Read the model definition and answer for the solid it produces. Units are mm, in the model's axes. A direction names the side the tool comes from. Coordinates: 2 decimals unless noted, no trailing zeros. Write each loop counter-clockwise with the first axis right and the second up, starting at its lowest first coordinate (ties: lowest second). Pieces come first, ordered by that corner, then holes. Notation, with made-up numbers: (74.5, 89) -> (90.5, 89) arc R12 ccw to (90.5, 103) -> close; hole circle Ø10 at (24, 57). An arc over 180 degrees is marked (long way). One line per item, written item: value. Start each with the question number.
from build123d import *

# Parameters (mm, degrees)
F0_W     = 25
F0_H     = 17
F1_DEPTH = 5.5
F3_DEPTH = 25
F5_DEPTH = 32.501
F7_DEPTH = 5.5
F9_DEPTH = 5.501


with BuildPart() as f1:
    # F0 (on Top) → F1 (new body)
    with BuildSketch(Plane.XY):
        with BuildLine():
            Line((-15.5, -24.3527164447), (15.5, -24.3527164447))
            Line((15.5, -24.3527164447), (15.5, 11.6472835553))
            Line((15.5, 11.6472835553), (16.5, 11.6472835553))
            ThreePointArc((16.5, 11.6472835553), (16.8535533906, 11.7937301647), (17, 12.1472835553))
            Line((17, 12.1472835553), (17, 16.843435978))
            ThreePointArc((17, 16.843435978), (16.8977774789, 17.6198931134), (16.5980762114, 18.343435978))
            Line((16.5980762114, 18.343435978), (15.1841674029, 20.7923978715))
            ThreePointArc((15.1841674029, 20.7923978715), (14.4494876631, 21.1305094363), (13.8862846459, 20.5500991403))
            Line((13.8862846459, 20.5500991403), (12.678607693, 12.7943144757))
            ThreePointArc((12.678607693, 12.7943144757), (12.5447185816, 11.6438227741), (12.5, 10.4864301451))
            Line((12.5, 10.4864301451), (12.5, 0.6472835553))
            ThreePointArc((12.5, 0.6472835553), (11.9142135624, -0.766930007), (10.5, -1.3527164447))
            Line((10.5, -1.3527164447), (5.7, -1.3527164447))
            ThreePointArc((5.7, -1.3527164447), (4.2857864376, -0.766930007), (3.7, 0.6472835553))
            Line((3.7, 0.6472835553), (3.7, 18.6472835553))
            ThreePointArc((3.7, 18.6472835553), (3.8975072906, 19.7178136174), (4.4640230758, 20.6473853514))
            Line((4.4640230758, 20.6473853514), (5.7959697488, 22.1364105755))
            ThreePointArc((5.7959697488, 22.1364105755), (6.362485534, 23.0659823095), (6.5599928246, 24.1365123716))
            Line((6.5599928246, 24.1365123716), (6.5599928246, 25.3001695988))
            ThreePointArc((6.5599928246, 25.3001695988), (6.2513345408, 25.762109365), (5.706439434, 25.6537229894))
            Line((5.706439434, 25.6537229894), (2.0786796564, 22.0259632118))
            ThreePointArc((2.0786796564, 22.0259632118), (1.4283614025, 21.0526931653), (1.2, 19.9046428682))
            Line((1.2, 19.9046428682), (1.2, -2.3527164447))
            Line((1.2, -2.3527164447), (-1.2, -2.3527164447))
            Line((-1.2, -2.3527164447), (-1.2, 20.1675462621))
            ThreePointArc((-1.2, 20.1675462621), (-1.4283614025, 21.3155965592), (-2.0786796564, 22.2888666056))
            Line((-2.0786796564, 22.2888666056), (-5.706439434, 25.9166263832))
            ThreePointArc((-5.706439434, 25.9166263832), (-6.2513345408, 26.0250127589), (-6.5599928246, 25.5630729926))
            Line((-6.5599928246, 25.5630729926), (-6.5599928246, 24.1365123716))
            ThreePointArc((-6.5599928246, 24.1365123716), (-6.362485534, 23.0659823095), (-5.7959697488, 22.1364105755))
            Line((-5.7959697488, 22.1364105755), (-4.4640230758, 20.6473853514))
            ThreePointArc((-4.4640230758, 20.6473853514), (-3.8975072906, 19.7178136174), (-3.7, 18.6472835553))
            Line((-3.7, 18.6472835553), (-3.7, 0.6472835553))
            ThreePointArc((-3.7, 0.6472835553), (-4.2857864376, -0.766930007), (-5.7, -1.3527164447))
            Line((-5.7, -1.3527164447), (-10.5, -1.3527164447))
            ThreePointArc((-10.5, -1.3527164447), (-11.9142135624, -0.766930007), (-12.5, 0.6472835553))
            Line((-12.5, 0.6472835553), (-12.5, 10.4864301451))
            ThreePointArc((-12.5, 10.4864301451), (-12.5447185816, 11.6438227741), (-12.678607693, 12.7943144757))
            Line((-12.678607693, 12.7943144757), (-13.8862846459, 20.5500991403))
            ThreePointArc((-13.8862846459, 20.5500991403), (-14.4494876631, 21.1305094363), (-15.1841674029, 20.7923978715))
            Line((-15.1841674029, 20.7923978715), (-16.5980762114, 18.343435978))
            ThreePointArc((-16.5980762114, 18.343435978), (-16.8977774789, 17.6198931134), (-17, 16.843435978))
            Line((-17, 16.843435978), (-17, 12.1472835553))
            ThreePointArc((-17, 12.1472835553), (-16.8535533906, 11.7937301647), (-16.5, 11.6472835553))
            Line((-16.5, 11.6472835553), (-15.5, 11.6472835553))
            Line((-15.5, 11.6472835553), (-15.5, -24.3527164447))
        make_face()
        with Locations((0, -12.8527164447)):
            Rectangle(F0_W, F0_H, mode=Mode.SUBTRACT)
    extrude(amount=F1_DEPTH)

    # F2 (on face) → F3 (join)
    with BuildSketch(Plane.YZ.offset(-12.5)):
        Polygon((-14.8527164447, 0), (-16.3527164447, 2.5980762114), (-17.8527164447, 0), align=None)
        with BuildLine():
            ThreePointArc((-6.8527164447, 1.5), (-9.4133766164, 2.5606601718), (-8.3527164447, 0))
            ThreePointArc((-8.3527164447, 0), (-7.2920562729, 0.4393398282), (-6.8527164447, 1.5))
        make_face()
    extrude(amount=F3_DEPTH)

    # F4 (on face) → F5 (cut, through all)
    with BuildSketch(Plane.YZ.offset(15.5)):
        Polygon((-24.3527164447, 0), (-21.3527164447, 0), (-24.3527164447, 3), align=None)
    extrude(amount=-F5_DEPTH, mode=Mode.SUBTRACT)



with BuildPart() as f7:
    # F6 (on face) → F7 (new body, through all)
    with BuildSketch(Plane.XY.offset(5.5)):
        with BuildLine():
            Line((17, -3.8527164447), (15.5, -3.8527164447))
            Line((15.5, -3.8527164447), (15.5, -21.3527164447))
            Line((15.5, -21.3527164447), (17, -21.3527164447))
            ThreePointArc((17, -21.3527164447), (17.7071067812, -21.0598232258), (18, -20.3527164447))
            Line((18, -20.3527164447), (18, -4.8527164447))
            ThreePointArc((18, -4.8527164447), (17.7071067812, -4.1456096635), (17, -3.8527164447))
        make_face()
    extrude(amount=-F7_DEPTH)

    # F8 (on face) → F9 (cut, through all)
    with BuildSketch(Plane.XY.offset(5.5)):
        Polygon((18, -6.3527164447), (18, -4.8527164447), (16.7009618943, -5.6027164447), align=None)
        Polygon((18, -21.3527164447), (18, -19.8527164447), (16.7009618943, -20.6027164447), align=None)
        Polygon((18, -19.8527164447), (18, -18.3527164447), (16.7009618943, -19.1027164447), align=None)
        Polygon((18, -18.3527164447), (18, -16.8527164447), (16.7009618943, -17.6027164447), align=None)
        Polygon((18, -16.8527164447), (18, -15.3527164447), (16.7009618943, -16.1027164447), align=None)
        Polygon((18, -15.3527164447), (18, -13.8527164447), (16.7009618943, -14.6027164447), align=None)
        Polygon((18, -13.8527164447), (18, -12.3527164447), (16.7009618943, -13.1027164447), align=None)
        Polygon((18, -12.3527164447), (18, -10.8527164447), (16.7009618943, -11.6027164447), align=None)
        Polygon((18, -10.8527164447), (18, -9.3527164447), (16.7009618943, -10.1027164447), align=None)
        Polygon((18, -9.3527164447), (18, -7.8527164447), (16.7009618943, -8.6027164447), align=None)
        Polygon((18, -7.8527164447), (18, -6.3527164447), (16.7009618943, -7.1027164447), align=None)
    extrude(amount=-F9_DEPTH, mode=Mode.SUBTRACT)


with BuildPart() as f1_1:
    add(f1.part)

    add(f7.part)  # F11 merges F7
    # F11: F7 across plane
    add(f7.part.mirror(Plane(origin=(0, -5.9573676074, 2.7906976744), x_dir=(0, 1, 0), z_dir=(1, 0, 0))))


solid = f1_1.part
1. A cutting plane is placed at C-C on y = 13.5. Give the vertices of the cut face in (x, z).
2. For a pull along Y with two mould halves and no side action, classify faces 1 (the face through (-12.543, 11.628, 2.712)), 2 (the face through (-15.5, 4, 3)), 3 (the face through (-17, 15, 3)) as +Y half, -Y half, draft (parallel to the pull), parting line (faces both ways), or undercut.
3. A cutting plane is placed at A-A on y = 8. Give the vertices of the cut face in (x, z).
4. Given pin 1 (2 mm diameter, centred on y = -3.5, z = 1, fed in from -X); pin 2 (2.5 mm diameter, centred on x = 7.5, z = 3, fed in from +Y); pin 3 (1.5 mm diameter, centred on x = 8, y = -1.5, fed in from -Z); pin 4 (0.8 mm diameter, centred on x = -16, z = 2.5, fed in from +Y), each flat-ended and moving along its own axis, determine where each tip first touches the part or whether it passes through.
5. A tool of negligible diameter and unlimited length cuts with its end or side. For faces 4 (the face through (0, -24.353, 4)), 5 (the face through (17.71, -4.15, 2.79)), 6 (the face through (16, -3.853, 3)), 7 (the face through (-4.27, -0.75, 2.71)), 8 (the face through (-13.274, 16.618, 2.712)), from which of +Z, -Z, +X, -X, +Y, -Y can it reach the whole face along a straight path? Write none if from no direction.
6. Find the intervals of material crossed by probe 1 along X at (y, z) = (5, 4.15); probe 2 along Y at (x, z) = (4, 2.05); probe 3 along Y at (x, z) = (-8.5, 0.85), in increasing order. Write a range as from..to.
7. A cutting plane is placed at B-B on x = 8.5. Give the vertices of the cut face in (y, z), then the cut area to 3 significant figures.
Derived:
1. outline: (-17, 0) -> (-12.79, 0) -> (-12.79, 5.5) -> (-17, 5.5) -> close; (-3.7, 0) -> (-1.2, 0) -> (-1.2, 5.5) -> (-3.7, 5.5) -> close; (1.2, 0) -> (3.7, 0) -> (3.7, 5.5) -> (1.2, 5.5) -> close; (12.79, 0) -> (17, 0) -> (17, 5.5) -> (12.79, 5.5) -> close
2. face 1: +Y half
2. face 2: undercut
2. face 3: draft
3. outline: (-15.5, 0) -> (-12.5, 0) -> (-12.5, 5.5) -> (-15.5, 5.5) -> close; (-3.7, 0) -> (-1.2, 0) -> (-1.2, 5.5) -> (-3.7, 5.5) -> close; (1.2, 0) -> (3.7, 0) -> (3.7, 5.5) -> (1.2, 5.5) -> close; (12.5, 0) -> (15.5, 0) -> (15.5, 5.5) -> (12.5, 5.5) -> close
4. pin 1: stops at x = -17.94
4. pin 2: stops at y = 25.76
4. pin 3: stops at z = 0
4. pin 4: stops at y = 20.07
5. face 4: +Z, -Z, +X, -X, -Y
5. face 5: +Z, -Z, +X, +Y
5. face 6: +Z, -Z, +X
5. face 7: +Z, -Z
5. face 8: +Z, -Z, +Y
6. probe 1: x = -15.5..-12.5, -3.7..-1.2, 1.2..3.7, 12.5..15.5
6. probe 2: y = -23.4..-21.35, -16.67..-16.04, -9.75..-6.96, -4.35..-0.41, 19.95..23.95
6. probe 3: y = -22.2..-21.35, -17.36..-15.34, -9.7..-7, -4.35..-1.35
7. outline: (-24.35, 3) -> (-21.35, 0) -> (-21.35, 5.5) -> (-24.35, 5.5) -> close; (-17.85, 0) -> (-14.85, 0) -> (-16.35, 2.6) -> close; circle Ø3 at (-8.35, 1.5); (-4.35, 0) -> (-1.35, 0) -> (-1.35, 5.5) -> (-4.35, 5.5) -> close
7. area: 39.5 mm2
